Geometry: final body of the model. Coordinates: model frame, mm. Round coordinates to 2 decimals unless told otherwise and drop trailing zeros. Loops run counter-clockwise (first coordinate to the right, second up) from the corner with the lowest first, then second, coordinate; pieces in that order, holes last. Notation, with made-up numbers: (47.5, 3.5) - (60.5, 3.5) arc R20 cw to (60.5, 11.5) - close; hole circle Ø7 at (15, 20). An arc over 180 degrees is marked (long way). Return JSON: item names as keys, results as strings. Group by question number.
1. Section B-B on z = 27.5. Return loops of the section in (x, y).
2. Section C-C on y = -21.75. Return loops of the section in (x, z).
3. Section A-A on x = -102.5. Return loops of the section in (y, z), and give its area (3 significant figures).
4. Material intervals for probe 1 along X at (y, z) = (-21.75, 44); probe 2 along X at (y, z) = (-1, 28.5); probe 3 along Z at (x, y) = (-89.5, -24), sorted ascending.
from build123d import *

# Parameters (mm, degrees)
F0_W     = 57.070940733
F0_H     = 62.6132022589
F1_DEPTH = 25.4
F0_W_2   = 13.6159174144
F0_H_2   = 7.0780348033
F3_SIZE  = 5.08


with BuildPart() as f1:
    # F0 (on Front) → F1 (new body)
    with BuildSketch(Plane.XZ):
        with Locations((-97.6289659739, 17.8792783991)):
            Rectangle(F0_W, F0_H)
    extrude(amount=F1_DEPTH)

    # F3
    f3_edges = [f1.edges().sort_by_distance(p)[0] for p in [
        (-97.628966, -25.4, 49.18588),
        (-126.164436, -25.4, 17.879278),
        (-97.628966, -25.4, -13.427323),
        (-69.093496, -25.4, 17.879278),
        (-97.628966, 0, 49.18588),
        (-126.164436, 0, 17.879278),
        (-97.628966, 0, -13.427323),
        (-69.093496, 0, 17.879278),
    ]]
    chamfer(f3_edges, length=F3_SIZE)


with BuildPart() as f1b:
    # F0 (on Front) → F1, piece 2 (new body)
    with BuildSketch(Plane.XZ):
        with Locations((-56.7812416703, -20.881687291)):
            Rectangle(F0_W_2, F0_H_2)
    extrude(amount=F1_DEPTH)


solid = f1.part
Taken from the geometry:
{
 "1": {"outline": "(-126.16, -20.32) - (-121.08, -25.4) - (-74.17, -25.4) - (-69.09, -20.32) - (-69.09, -5.08) - (-74.17, 0) - (-121.08, 0) - (-126.16, -5.08) - close"},
 "2": {"outline": "(-124.73, -12) - (-70.52, -12) - (-70.52, 47.76) - (-124.73, 47.76) - close"},
 "3": {"outline": "(-25.4, -8.35) - (-20.32, -13.43) - (-5.08, -13.43) - (0, -8.35) - (0, 44.11) - (-5.08, 49.19) - (-20.32, 49.19) - (-25.4, 44.11) - close", "area": "1,540 mm2"},
 "4": {"probe 1": "-124.73 to -70.52", "probe 2": "-122.08 to -73.17", "probe 3": "-9.75 to 45.51"}
}
